```python
from build123d import *

# Parameters (mm, degrees)
SKETCH_1_W          = 210
SKETCH_1_H          = 132
EXTRUDE_1_DEPTH     = 1
SKETCH_3_W          = 1
SKETCH_3_H          = 132
EXTRUDE_2_DEPTH     = 81
SKETCH_2_R          = 1.5
CUT_EXTRUDE_1_DEPTH = 1
SKETCH_4_R          = 1.5
CUT_EXTRUDE_2_DEPTH = 211


with BuildPart() as part:
    # 草图1 → 凸台-拉伸1 (new body)
    with BuildSketch(Plane.XY):
        Rectangle(SKETCH_1_W, SKETCH_1_H)
    extrude(amount=EXTRUDE_1_DEPTH)

    # 草图3 → 凸台-拉伸2 (add)
    with BuildSketch(Plane.XY.offset(1)):
        with Locations((104.5, 0)):
            Rectangle(SKETCH_3_W, SKETCH_3_H)
    extrude(amount=EXTRUDE_2_DEPTH)

    # 草图2 → 切除-拉伸1 (cut)
    with BuildSketch(Plane.XY.offset(1)):
        with Locations((-75, 63)):
            Circle(SKETCH_2_R)
        with Locations((75, 63)):
            Circle(SKETCH_2_R)
        with Locations((75, -63)):
            Circle(SKETCH_2_R)
        with Locations((-75, -63)):
            Circle(SKETCH_2_R)
    extrude(amount=-CUT_EXTRUDE_1_DEPTH, mode=Mode.SUBTRACT)

    # 草图4 → 切除-拉伸2 (cut, through all)
    with BuildSketch(Plane(origin=(105, 0, 0), x_dir=(0, 0, -1), z_dir=(1, 0, 0))):
        with Locations((-41, 63)):
            Circle(SKETCH_4_R)
        with Locations((-41, -63)):
            Circle(SKETCH_4_R)
    extrude(amount=-CUT_EXTRUDE_2_DEPTH, mode=Mode.SUBTRACT)


solid = part.part
```
Geometry check sheet. Reference: the model listing, model coordinates, mm. A direction names the side the tool comes from. Give positions to 0.01 mm unless a question says otherwise; leave off trailing zeros. Loops run counter-clockwise (first coordinate to the right, second up) from the corner with the lowest first, then second, coordinate; pieces in that order, holes last. Notation, with made-up numbers: M 35,-15 L 70,-15 A26 cw 70,2 Z; hole C 68.25,4 d11. An arc over 180 degrees is marked long. Write item = value, one per line. Start each with the question number.
1. Section check B-B, the plane z = 70. Enter the section's corners in (x, y).
2. Section check C-C, the plane x = -11.5. Enter the section's corners in (y, z), plus the area to 3 significant figures.
3. Tool access check on faces 1 (the face through (104, -1, 41)), 2 (the face through (105, -1, 40)). Record the directions out of +Z, -Z, +X, -X, +Y, -Y that give a thin tool (end or side, any length) a straight path to the whole face; none if there is none.
4. Go/stop test with flat-tipped pins: P1, Ø8, axis at x = -40.5, y = 25, coming from the +Z side; P2, Ø12, axis at y = -5.5, z = 31.5, coming from the -X side. Record where each tip stops, or that it passes through.
5. Thickness scan on probe 1 along Y at (x, z) = (104.25, 41); probe 2 along X at (y, z) = (44, 41); probe 3 along Z at (x, y) = (89.5, 21.5). Record the ranges inside material, lowest first.
6. Section check A-A, the plane y = 26. Enter the section's corners in (x, z).
Values follow:
q1.outline = M 104,-66 L 105,-66 L 105,66 L 104,66 Z
q2.outline = M -66,0 L 66,0 L 66,1 L -66,1 Z
q2.area = 132 mm^2
q3.face_1 = +Z, -X, +Y, -Y
q3.face_2 = +Z, -Z, +X, +Y, -Y
q4.P1 = 1
q4.P2 = 104
q5.probe_1 = -66 to -64.5, -61.5 to 61.5, 64.5 to 66
q5.probe_2 = 104 to 105
q5.probe_3 = 0 to 1
q6.outline = M -105,0 L 105,0 L 105,82 L 104,82 L 104,1 L -105,1 Z
